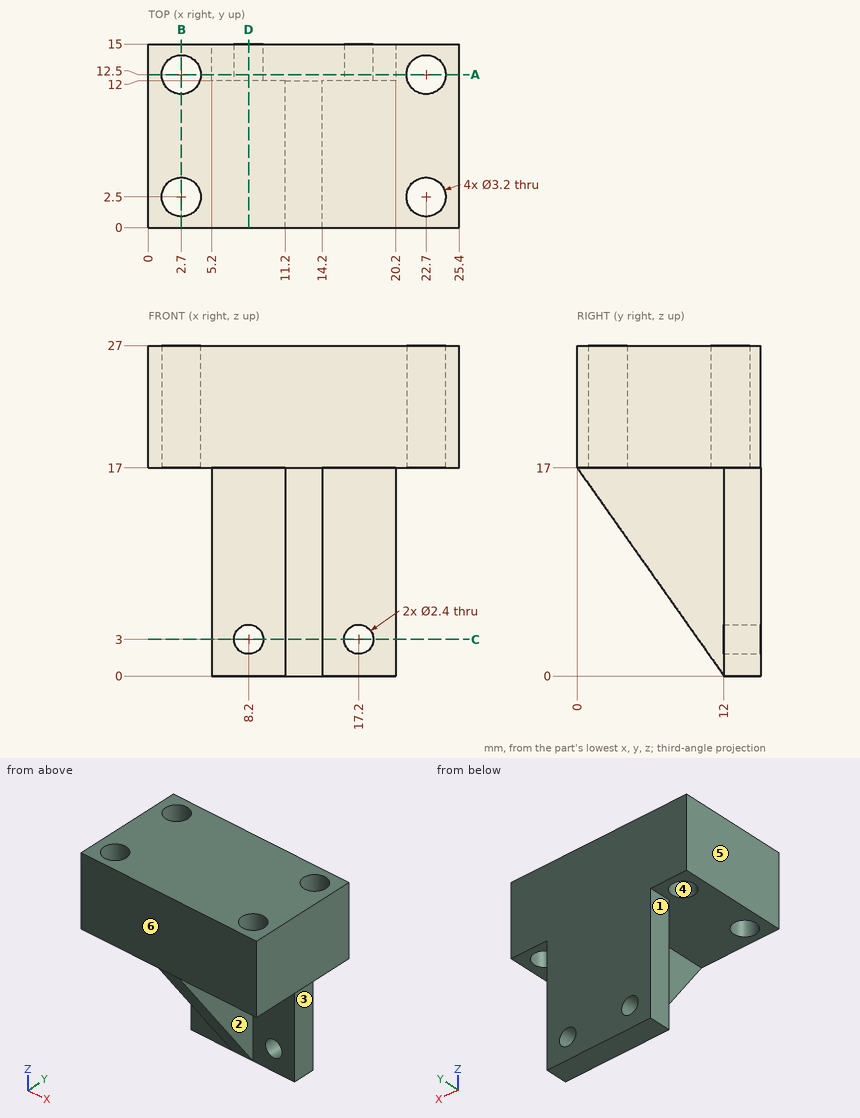
Could you check a few things on this drawing? It's one solid part, dimensions in mm from its lowest x, y, z. A direction names the side the tool comes from. Give positions to 0.01 mm unless a question says otherwise; leave off trailing zeros. Write each loop counter-clockwise with the first axis right and the second up, starting at its lowest first coordinate (ties: lowest second). Pieces come first, ordered by that corner, then holes. Notation, with made-up numbers: (43.25, 3.5) -> (92.25, 3.5) arc R28 cw to (92.25, 27.5) -> close; hole circle Ø1 at (3.25, 78.5). An arc over 180 degrees is marked (long way). Write item = value, one per line.
(1) I need wall thicknesses on probe 1 along X at (y, z) = (2.5, 21.25); probe 2 along Y at (x, z) = (2.7, 21.75); probe 3 along Z at (x, y) = (17.2, 13.7). Which ranges of each line are inside material? Lowest first, please. Write a range as from..to.
Worked out:
probe_1 = 0..1.1, 4.3..21.1, 24.3..25.4
probe_2 = 0..0.9, 4.1..10.9, 14.1..15
probe_3 = 0..1.8, 4.2..27
(2) Suppose I cut it at A-A on y = 12.5. Write out the boundary of the cut face in (x, z).
Worked out:
outline = (0, 17) -> (1.1, 17) -> (1.1, 27) -> (0, 27) -> close; (4.3, 17) -> (5.2, 17) -> (5.2, 0) -> (20.2, 0) -> (20.2, 17) -> (21.1, 17) -> (21.1, 27) -> (4.3, 27) -> close; (24.3, 17) -> (25.4, 17) -> (25.4, 27) -> (24.3, 27) -> close; hole circle Ø2.4 at (8.2, 3); hole circle Ø2.4 at (17.2, 3)
(3) Thinking about a two-plate mould opening in Y: for the marked faces 4, 5 and 6, which applies, released by +Y, released by -Y, zero draft, split by the parting line, or undercut?
Worked out:
face_4 = undercut
face_5 = zero draft
face_6 = released by -Y
(4) Suppose I cut it at B-B on x = 2.7. Write out the boundary of the cut face in (y, z), then the cut area to 3 significant figures.
Worked out:
outline = (0, 17) -> (0.9, 17) -> (0.9, 27) -> (0, 27) -> close; (4.1, 17) -> (10.9, 17) -> (10.9, 27) -> (4.1, 27) -> close; (14.1, 17) -> (15, 17) -> (15, 27) -> (14.1, 27) -> close
area = 86.0 mm^2
(5) Suppose I cut it at D-D on x = 8.2. Write out the boundary of the cut face in (y, z), then the cut area to 3 significant figures.
Worked out:
outline = (0, 17) -> (12, 17) -> (12, 4.2) -> (15, 4.2) -> (15, 27) -> (0, 27) -> close; (12, 0) -> (15, 0) -> (15, 1.8) -> (12, 1.8) -> close
area = 194 mm^2
(6) Suppose I cut it at C-C on z = 3. Write out the boundary of the cut face in (x, y).
Worked out:
outline = (5.2, 12) -> (7, 12) -> (7, 15) -> (5.2, 15) -> close; (9.4, 12) -> (11.2, 12) -> (11.2, 9.88) -> (14.2, 9.88) -> (14.2, 12) -> (16, 12) -> (16, 15) -> (9.4, 15) -> close; (18.4, 12) -> (20.2, 12) -> (20.2, 15) -> (18.4, 15) -> close
(7) I'm going to push flat-ended pins straight in: P1, Ø4, axis at x = 2.7, y = 2.5, coming from the -Z side; P2, Ø2, axis at x = 19.5, z = 10.5, coming from the -Y side; P3, Ø3.5, axis at y = 6.5, z = 9.5, coming from the +X side. Where does each tip first touch, or does it pass through?
Worked out:
P1 = 17
P2 = 12
P3 = 14.2
(8) For the marked faces 1, 2 and 3, which set-ups out of +Z, -Z, +X, -X, +Y, -Y let a thin tool reach every point of the face, with its end or its side?
Worked out:
face_1 = -Z, -X, +Y, -Y
face_2 = -Z, +X, -Y
face_3 = -Z, +X, +Y, -Y
